from build123d import *

# Parameters (mm, degrees)
SKETCH_1_W                       = 62
SKETCH_1_H                       = 38
SM_BASE_FLANGE_1_DEPTH           = 2
SM_EDGE_FLANGE_1_STRIP_W         = 9.4732
SM_EDGE_FLANGE_1_STRIP_H         = 2
SM_EDGE_FLANGE_1_STRIP_CUT_DEPTH = 38
SM_EDGE_FLANGE_1_DEPTH           = 38
SM_START                         = 2
SM_EDGE_FLANGE_1_PROFILE_W       = 38
SM_EDGE_FLANGE_1_PROFILE_H       = 56.7366
SM_EDGE_FLANGE_1_PROFILE_R       = 12.668336417
SM_EDGE_FLANGE_1_FLAT_DEPTH      = 2


# Sheet-metal steps are written as plain solids
with BuildPart() as part:
    # Sketch 1 → 基材-凸緣1 (new body)
    with BuildSketch(Plane(origin=(0, 0, 0), x_dir=(1, 0, 0), z_dir=(0, 1, 0))):
        Rectangle(SKETCH_1_W, SKETCH_1_H)
    extrude(amount=SM_BASE_FLANGE_1_DEPTH)

    # 邊線-凸緣1 strip (across the edge) → 邊線-凸緣1 strip cut (cut)
    with BuildSketch(Plane(origin=(31, 2, 19), x_dir=(-1, 0, 0), z_dir=(0, 0, -1))):
        with Locations((-4, -1)):
            Rectangle(SM_EDGE_FLANGE_1_STRIP_W, SM_EDGE_FLANGE_1_STRIP_H)
    extrude(amount=SM_EDGE_FLANGE_1_STRIP_CUT_DEPTH, mode=Mode.SUBTRACT)

    # 邊線-凸緣1 bend section (across the edge) → 邊線-凸緣1 (add)
    with BuildSketch(Plane(origin=(31, 2, 19), x_dir=(-1, 0, 0), z_dir=(0, 0, -1))):
        with BuildLine():
            Line((-2, 0.7366), (0, 0.7366))
            ThreePointArc((0, 0.7366), (0.215745145, 0.215745145), (0.7366, 0))
            Line((0.7366, 0), (0.7366, -2))
            ThreePointArc((0.7366, -2), (-1.198468417, -1.198468417), (-2, 0.7366))
        make_face()
    extrude(amount=SM_EDGE_FLANGE_1_DEPTH)

    # 邊線-凸緣1 profile (on flange) → 邊線-凸緣1 flat (add)
    with BuildSketch(Plane(origin=(31, 2, 0), x_dir=(0, 0, -1), z_dir=(1, 0, 0)).offset(SM_START)):
        with Locations((0, 29.1049)):
            Rectangle(SM_EDGE_FLANGE_1_PROFILE_W, SM_EDGE_FLANGE_1_PROFILE_H)
        with Locations((0, 28.7366)):
            Circle(SM_EDGE_FLANGE_1_PROFILE_R, mode=Mode.SUBTRACT)
    extrude(amount=-SM_EDGE_FLANGE_1_FLAT_DEPTH)


solid = part.part
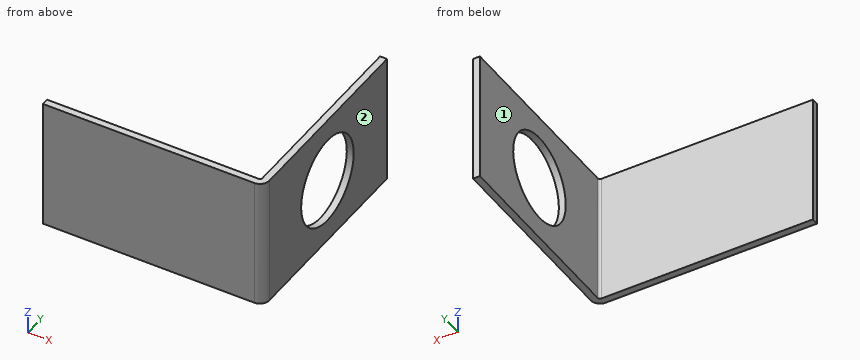
Can you work these out from the model? Positions are in its coordinate system, mm. Face numbers are marked on the shaded views. A direction names the side the tool comes from. Coordinates: 2 decimals unless noted, no trailing zeros. Write each loop counter-clockwise with the first axis right and the second up, starting at its lowest first coordinate (ties: lowest second). Pieces come first, ordered by that corner, then holes. Notation, with made-up numbers: (41, 63.25) -> (99, 63.25) arc R15 cw to (99, 69.25) -> close; hole circle Ø2 at (-13, 80.5). An arc over 180 degrees is marked (long way). Write each question's results on one line, items separated by ' | '. Start each with the question number.
Item 1: On a 3-axis mill with a long thin cutter (end or side, diameter ignored), from which of +Z, -Z, +X, -X, +Y, -Y can I reach the whole of each face in a straight line? I mean the marked faces 1 and 2. Say none if no direction works.
Item 2: If we section it at D-D, the plane x = -5: Write out the boundary of the cut face in (y, z).
Item 3: I'm going to push flat-ended pins straight in: P1, Ø5, axis at y = 8.5, z = 1.5, coming from the -X side; P2, Ø10, axis at x = -11, z = -1.5, coming from the +Y side; P3, Ø5, axis at x = -8, z = 12.5, coming from the -Y side. Where does each tip first touch, or does it pass through?
Item 4: If we section it at B-B, the plane z = 15.5: Write out the boundary of the cut face in (x, y).
Item 5: If we section it at C-C, the plane y = 54.5: Write out the boundary of the cut face in (x, z).
Item 6: Please list where these lines run through material, in increasing order: probe 1 along Y at (x, z) = (23.5, 11); probe 2 along X at (y, z) = (17.5, -0.5); probe 3 along Y at (x, z) = (32, 0).
Item 7: If we section it at A-A, the plane z = 0: Write out the boundary of the cut face in (x, y), and give its area (3 significant figures).
Answer block:
1) face 1: +Z, -Z, -X, +Y | face 2: +Z, -Z, +X, +Y, -Y
2) outline: (0, -19) -> (2, -19) -> (2, 19) -> (0, 19) -> close
3) P1: x = 31 | P2: y = 2 | P3: y = 0
4) outline: (-31, 0) -> (30.26, 0) arc R2.74 ccw to (33, 2.74) -> (33, 59.47) -> (31, 59.47) -> (31, 2.74) arc R0.74 cw to (30.26, 2) -> (-31, 2) -> close
5) outline: (31, -19) -> (33, -19) -> (33, 19) -> (31, 19) -> close
6) probe 1: 0 to 2 | probe 2: 31 to 33 | probe 3: 0.62 to 18.07, 43.4 to 59.47
7) outline: (-31, 0) -> (30.26, 0) arc R2.74 ccw to (33, 2.74) -> (33, 18.07) -> (31, 18.07) -> (31, 2.74) arc R0.74 cw to (30.26, 2) -> (-31, 2) -> close; (31, 43.4) -> (33, 43.4) -> (33, 59.47) -> (31, 59.47) -> close | area: 191 mm²
